Build history of the part. All positions in model axes, mm. A direction names the side the tool comes from. Coordinates: 2 decimals unless noted, no trailing zeros. Write each loop counter-clockwise with the first axis right and the second up, starting at its lowest first coordinate (ties: lowest second). Pieces come first, ordered by that corner, then holes.
```python
from build123d import *

# Parameters (mm, degrees)
F0_R     = 2.75
F0_W     = 4
F0_H     = 10
F0_W_2   = 6
F0_H_2   = 8
F1_DEPTH = 10.5
F0_R_2   = 2.5
F2_DEPTH = 3
F3_DEPTH = 1


with BuildPart() as f1:
    # F0 (on Top) → F1 (new body)
    with BuildSketch(Plane.XY):
        with BuildLine():
            Line((-20, -13.5), (-9.5, -13.5))
            Line((-9.5, -13.5), (-9.5, -5.5))
            Line((-9.5, -5.5), (-13, -5.5))
            Line((-13, -5.5), (-13, -1.5))
            Line((-13, -1.5), (-9.5, -1.5))
            Line((-9.5, -1.5), (-9.5, 3.9896013553))
            ThreePointArc((-9.5, 3.9896013553), (-10.75, 7), (-9.5, 10.0103986447))
            Line((-9.5, 10.0103986447), (-9.5, 13.5))
            Line((-9.5, 13.5), (-20, 13.5))
            Line((-20, 13.5), (-20, -13.5))
        make_face()
        with Locations((-16, -9.5)):
            Circle(F0_R, mode=Mode.SUBTRACT)
        with BuildLine():
            Line((-3.5, 10.0103986447), (-3.5, 13.5))
            Line((-3.5, 13.5), (-9.5, 13.5))
            Line((-9.5, 13.5), (-9.5, 10.0103986447))
            ThreePointArc((-9.5, 10.0103986447), (-6.5, 11.25), (-3.5, 10.0103986447))
        make_face()
        with BuildLine():
            Line((-3.5, -13.5), (20, -13.5))
            Line((20, -13.5), (20, 13.5))
            Line((20, 13.5), (-3.5, 13.5))
            Line((-3.5, 13.5), (-3.5, 10.0103986447))
            ThreePointArc((-3.5, 10.0103986447), (-2.574920383, 8.6298006013), (-2.25, 7))
            ThreePointArc((-2.25, 7), (-2.574920383, 5.3701993987), (-3.5, 3.9896013553))
            Line((-3.5, 3.9896013553), (-3.5, -1.5))
            Line((-3.5, -1.5), (0, -1.5))
            Line((0, -1.5), (0, -5.5))
            Line((0, -5.5), (-3.5, -5.5))
            Line((-3.5, -5.5), (-3.5, -13.5))
        make_face()
        with Locations((3, -9.5)):
            Circle(F0_R, mode=Mode.SUBTRACT)
        with Locations((9.5, -4)):
            Rectangle(F0_W, F0_H, mode=Mode.SUBTRACT)
        with Locations((-6.5, -9.5)):
            Rectangle(F0_W_2, F0_H_2)
        with BuildLine():
            Line((-9.5, -1.5), (-3.5, -1.5))
            Line((-3.5, -1.5), (-3.5, 3.9896013553))
            ThreePointArc((-3.5, 3.9896013553), (-6.5, 2.75), (-9.5, 3.9896013553))
            Line((-9.5, 3.9896013553), (-9.5, -1.5))
        make_face()
    extrude(amount=F1_DEPTH)

    # F0 (on Top) → F2 (join)
    with BuildSketch(Plane.XY):
        with BuildLine():
            Line((-9.5, 3.9896013553), (-9.5, 10.0103986447))
            ThreePointArc((-9.5, 10.0103986447), (-10.75, 7), (-9.5, 3.9896013553))
        make_face()
        with BuildLine():
            Line((-3.5, 3.9896013553), (-3.5, 10.0103986447))
            ThreePointArc((-3.5, 10.0103986447), (-6.5, 11.25), (-9.5, 10.0103986447))
            Line((-9.5, 10.0103986447), (-9.5, 3.9896013553))
            ThreePointArc((-9.5, 3.9896013553), (-6.5, 2.75), (-3.5, 3.9896013553))
        make_face()
        with Locations((-6.5, 7)):
            Circle(F0_R_2, mode=Mode.SUBTRACT)
        with BuildLine():
            ThreePointArc((-2.25, 7), (-2.574920383, 8.6298006013), (-3.5, 10.0103986447))
            Line((-3.5, 10.0103986447), (-3.5, 3.9896013553))
            ThreePointArc((-3.5, 3.9896013553), (-2.574920383, 5.3701993987), (-2.25, 7))
        make_face()
    extrude(amount=F2_DEPTH)

    # F0 (on Top) → F3 (join)
    with BuildSketch(Plane.XY):
        with BuildLine():
            Line((-3.5, 10.0103986447), (-3.5, 13.5))
            Line((-3.5, 13.5), (-9.5, 13.5))
            Line((-9.5, 13.5), (-9.5, 10.0103986447))
            ThreePointArc((-9.5, 10.0103986447), (-6.5, 11.25), (-3.5, 10.0103986447))
        make_face()
        with BuildLine():
            Line((-3.5, 3.9896013553), (-3.5, 10.0103986447))
            ThreePointArc((-3.5, 10.0103986447), (-6.5, 11.25), (-9.5, 10.0103986447))
            Line((-9.5, 10.0103986447), (-9.5, 3.9896013553))
            ThreePointArc((-9.5, 3.9896013553), (-6.5, 2.75), (-3.5, 3.9896013553))
        make_face()
        with Locations((-6.5, 7)):
            Circle(F0_R_2, mode=Mode.SUBTRACT)
        with BuildLine():
            Line((-9.5, -1.5), (-3.5, -1.5))
            Line((-3.5, -1.5), (-3.5, 3.9896013553))
            ThreePointArc((-3.5, 3.9896013553), (-6.5, 2.75), (-9.5, 3.9896013553))
            Line((-9.5, 3.9896013553), (-9.5, -1.5))
        make_face()
        with Locations((-6.5, -9.5)):
            Rectangle(F0_W_2, F0_H_2)
    extrude(amount=-F3_DEPTH)


solid = f1.part
```
1. Probe line 1 along Y through (x, z) = (-6.5, 1.2); line 2 along X through (y, z) = (-4.5, 9.75); line 3 along X through (y, z) = (-0.5, 2.25). List the from-to ranges inside material, lowest first.
Computed values:
line 1: y = -13.5 to -5.5, -1.5 to 4.5, 9.5 to 13.5
line 2: x = -20 to -13, 0 to 7.5, 11.5 to 20
line 3: x = -20 to 7.5, 11.5 to 20
2. Saw through at C-C on y = -9.5. List the corners of the cut face in (x, z), plus the area to 4 significant figures.
Computed values:
outline: (-20, 0) - (-18.75, 0) - (-18.75, 10.5) - (-20, 10.5) - close; (-13.25, 0) - (-9.5, 0) - (-9.5, -1) - (-3.5, -1) - (-3.5, 0) - (0.25, 0) - (0.25, 10.5) - (-13.25, 10.5) - close; (5.75, 0) - (20, 0) - (20, 10.5) - (5.75, 10.5) - close
area: 310.5 mm2
3. Mould opens along Y. For faces 6 (the face through (9, -9, 5)), 7 (the face through (-3.5, 5.9, -0.5)), 8 (the face through (0, 13.5, 5)) say: +Y half, -Y half, draft (parallel to the pull), parting line (faces both ways), or undercut.
Computed values:
face 6: undercut
face 7: draft
face 8: +Y half
4. Flat gauge pins, fed straight in: pin 1 (0.5 mm diameter, centred on y = 7, z = -0.5, fed in from +X); pin 2 (0.5 mm diameter, centred on y = -9, z = -0.5, fed in from -X); pin 3 (6.5 mm diameter, centred on x = -6.5, y = 7, fed in from +Z). Where does each tip first touch, or does it go through?
Computed values:
pin 1: stops at x = -3.5
pin 2: stops at x = -9.5
pin 3: stops at z = 3
5. Saw through at D-D on y = 2. List the corners of the cut face in (x, z).
Computed values:
outline: (-20, 0) - (-9.5, 0) - (-9.5, -1) - (-3.5, -1) - (-3.5, 0) - (20, 0) - (20, 10.5) - (-20, 10.5) - close
6. 3-axis set-ups, long thin cutter, end or side, ignore diameter. For faces 1 (the face through (8, 3, 0)), 2 (the face through (0, -3, 5)), 3 (the face through (20, 0, 5)), 4 (the face through (-9.5, -9.6, -0.5)), 5 (the face through (-7, -9, -1)): which of +Z, -Z, +X, -X, +Y, -Y reach the whole face in a straight line?
Computed values:
face 1: -Z, +X, +Y, -Y
face 2: +Z, -Z
face 3: +Z, -Z, +X, +Y, -Y
face 4: -Z, -X, +Y, -Y
face 5: -Z, +X, -X, +Y, -Y
7. Saw through at A-A on x = 3. List the corners of the cut face in (y, z).
Computed values:
outline: (-13.5, 0) - (-12.25, 0) - (-12.25, 10.5) - (-13.5, 10.5) - close; (-6.75, 0) - (13.5, 0) - (13.5, 10.5) - (-6.75, 10.5) - close
8. Saw through at B-B on z = 3.5. List the corners of the cut face in (x, y).
Computed values:
outline: (-20, -13.5) - (20, -13.5) - (20, 13.5) - (-20, 13.5) - close; hole circle Ø5.5 at (-16, -9.5); hole (-13, -5.5) - (0, -5.5) - (0, -1.5) - (-13, -1.5) - close; hole circle Ø8.5 at (-6.5, 7); hole circle Ø5.5 at (3, -9.5); hole (7.5, -9) - (11.5, -9) - (11.5, 1) - (7.5, 1) - close
